The model under review builds one solid part; all positions refer to its coordinate system, in mm. A direction names the side the tool comes from. Give positions to 0.01 mm unless a question says otherwise; leave off trailing zeros. Write each loop counter-clockwise with the first axis right and the second up, starting at its lowest first coordinate (ties: lowest second). Pieces come first, ordered by that corner, then holes.
from build123d import *

# Parameters (mm, degrees)
F1_DEPTH = 15
F2_R     = 8
F3_DEPTH = 15.001
F4_R     = 10
F5_R     = 5
F6_R     = 5
F7_R     = 5


with BuildPart() as f1:
    # F0 (on Front) → F1 (new body)
    with BuildSketch(Plane.XZ):
        Polygon((50.351163, 50), (-64.648837, 50), (-64.648837, 0), (-89.648837, 0), (-89.648837, -20), (-49.648837, -20), (-49.648837, 35), (35.351163, 35), (35.351163, 0), (10.351163, 0), (10.351163, -20), (50.351163, -20), align=None)
    extrude(amount=F1_DEPTH)

    # F2 (on face) → F3 (cut, through all)
    with BuildSketch(Plane.XZ.offset(15)):
        with Locations((-72.648837, 0)):
            Circle(F2_R)
        with Locations((27.351163, 0)):
            Circle(F2_R)
    extrude(amount=-F3_DEPTH, mode=Mode.SUBTRACT)

    # F4
    f4_edges = [f1.edges().sort_by_distance(p)[0] for p in [
        (-64.648837, -7.5, 50),
        (50.351163, -7.5, 50),
    ]]
    fillet(f4_edges, radius=F4_R)

    # F5
    f5_edges = [f1.edges().sort_by_distance(p)[0] for p in [
        (-89.648837, -7.5, 0),
        (10.351163, -7.5, 0),
        (-49.648837, -7.5, 35),
        (35.351163, -7.5, 35),
    ]]
    fillet(f5_edges, radius=F5_R)

    # F6
    f6_edges = [f1.edges().sort_by_distance(p)[0] for p in [
        (-89.648837, -7.5, -20),
        (10.351163, -7.5, -20),
    ]]
    fillet(f6_edges, radius=F6_R)

    # F7
    f7_edges = [f1.edges().sort_by_distance(p)[0] for p in [
        (-49.648837, -7.5, -20),
        (50.351163, -7.5, -20),
    ]]
    fillet(f7_edges, radius=F7_R)


solid = f1.part
1) Consider section A-A, the plane z = 18. Give the boundary of the cut face in (x, y).
2) Insertion check: pin 1 (3 mm diameter, centred on y = -1.5, z = -1, fed in from -X); pin 2 (4.5 mm diameter, centred on x = -82, y = -7.5, fed in from +Z); pin 3 (7.5 mm diameter, centred on y = -5, z = 8.5, fed in from -X). Each pin has a flat end and moves straight along its axis. Give the tip position at first contact, or say it passes through.
3) The part is to be moulded in two halves that separate along X. For faces 1 (the flat face through (35.351, -7, 15)), 2 (the flat face through (-49.649, -7, 7)), 3 (the flat face through (50.351, -7, 12)), 4 (the cylindrical face through (-88.15, -7.6, -18.57)), say which applies: +X half, -X half, draft (parallel to the pull), parting line (faces both ways), or undercut.
4) Tool access review of faces 5 (the cylindrical face through (-72.8, -7.6, -8)), 6 (the flat face through (-21, 0, 39)), 7 (the flat face through (-64.649, -7, 20)), 8 (the cylindrical face through (-51.075, -7.605, -18.496)), 9 (the flat face through (-8, -7, 35)): name each direction out of +Z, -Z, +X, -X, +Y, -Y from which nothing blocks a thin tool from reaching the whole face with its end or side.
5) Consider section C-C, the plane x = -9. Give the boundary of the cut face in (y, z).
6) Consider section B-B, the plane y = -9.5. Give the boundary of the cut face in (x, z).
7) To check wall thickness, follow probe 1 along X at (y, z) = (-6, 5); probe 2 along X at (y, z) = (-2, -10); probe 3 along X at (y, z) = (-7.5, 36). State the ranges of each line that lie inside material, in increasing order.
Answer block:
1. outline: (-64.65, -15) - (-49.65, -15) - (-49.65, 0) - (-64.65, 0) - close; (35.35, -15) - (50.35, -15) - (50.35, 0) - (35.35, 0) - close
2. pin 1: stops at x = -88.98
2. pin 2: stops at z = 0
2. pin 3: stops at x = -64.65
3. face 1: undercut
3. face 2: undercut
3. face 3: +X half
3. face 4: -X half
4. face 5: +Z, +Y, -Y
4. face 6: +Z, -Z, +X, -X, +Y
4. face 7: +Z, -X, +Y, -Y
4. face 8: -Z, +Y, -Y
4. face 9: +Y, -Y
5. outline: (-15, 35) - (0, 35) - (0, 50) - (-15, 50) - close
6. outline: (-89.65, -15) arc R5 ccw to (-84.65, -20) - (-54.65, -20) arc R5 ccw to (-49.65, -15) - (-49.65, 30) arc R5 cw to (-44.65, 35) - (30.35, 35) arc R5 cw to (35.35, 30) - (35.35, 0) arc R8 cw to (19.35, 0) - (15.35, 0) arc R5 ccw to (10.35, -5) - (10.35, -15) arc R5 ccw to (15.35, -20) - (45.35, -20) arc R5 ccw to (50.35, -15) - (50.35, 40) arc R10 ccw to (40.35, 50) - (-54.65, 50) arc R10 ccw to (-64.65, 40) - (-64.65, 0) arc R8 cw to (-80.65, 0) - (-84.65, 0) arc R5 ccw to (-89.65, -5) - close
7. probe 1: x = -64.65 to -49.65, 35.35 to 50.35
7. probe 2: x = -89.65 to -49.65, 10.35 to 50.35
7. probe 3: x = -64.65 to 50.35
